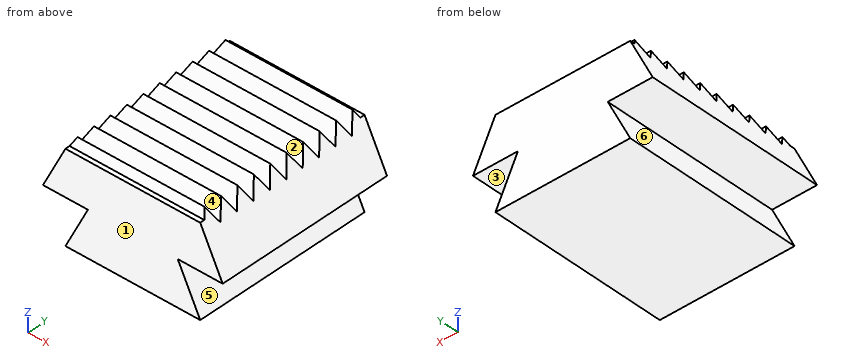
from build123d import *

# Parameters (mm, degrees)
BOSS_EXTRUDE1_DEPTH             = 5
BOSS_EXTRUDE1_DEPTH_BACK        = 5
BOSS_EXTRUDE2_REACH             = 10.66
BOSS_EXTRUDE2_DIRECTION_2_REACH = 10.66
CUT_EXTRUDE1_DEPTH              = 9.660254038
CUT_EXTRUDE1_DEPTH_BACK         = 9.660254038


with BuildPart() as part:
    # Sketch1 → Boss-Extrude1 (new, two sides: drawn at the far end of the back side and taken through both)
    with BuildSketch(Plane(origin=(0, 0, 0), x_dir=(1, 0, 0), z_dir=(0, 1, 0)).offset(-BOSS_EXTRUDE1_DEPTH_BACK)):
        Polygon((-3.75, 0), (3.75, 0), (5, 2.5), (2.5, 2.5), (3.75, 5), (-3.75, 5), (-2.5, 2.5), (-5, 2.5), align=None)
    extrude(amount=BOSS_EXTRUDE1_DEPTH + BOSS_EXTRUDE1_DEPTH_BACK)

    # Boss-Extrude2: up to this plane
    boss_extrude2_end = Plane(origin=(3.75, -5, 0), z_dir=(0.8944271909999159, 0, 0.44721359549995815))
    # Sketch3 → Boss-Extrude2 (add, up to the surface)
    with BuildSketch(Plane(origin=(0, 0, 0), x_dir=(0, 0, -1), z_dir=(1, 0, 0)), mode=Mode.PRIVATE) as boss_extrude2_sk1:
        Polygon((-0.433012702, 4.5), (0.216506351, 4.125), (0.216506351, 4.875), align=None)
    boss_extrude2_tool1 = split(extrude(boss_extrude2_sk1.sketch, amount=BOSS_EXTRUDE2_REACH, mode=Mode.PRIVATE), bisect_by=boss_extrude2_end, keep=Keep.BOTH, mode=Mode.PRIVATE)
    add(boss_extrude2_tool1.solids().sort_by_distance((0, 4.5, 0))[0])
    # Sketch3 → Boss-Extrude2 (add, up to the surface)
    with BuildSketch(Plane(origin=(0, 0, 0), x_dir=(0, 0, -1), z_dir=(1, 0, 0)), mode=Mode.PRIVATE) as boss_extrude2_sk2:
        Polygon((0.216506351, 3.875), (-0.433012702, 3.5), (0.216506351, 3.125), align=None)
    boss_extrude2_tool2 = split(extrude(boss_extrude2_sk2.sketch, amount=BOSS_EXTRUDE2_REACH, mode=Mode.PRIVATE), bisect_by=boss_extrude2_end, keep=Keep.BOTH, mode=Mode.PRIVATE)
    add(boss_extrude2_tool2.solids().sort_by_distance((0, 3.5, 0))[0])
    # Sketch3 → Boss-Extrude2 (add, up to the surface)
    with BuildSketch(Plane(origin=(0, 0, 0), x_dir=(0, 0, -1), z_dir=(1, 0, 0)), mode=Mode.PRIVATE) as boss_extrude2_sk3:
        Polygon((0.216506351, 2.875), (-0.433012702, 2.5), (0.216506351, 2.125), align=None)
    boss_extrude2_tool3 = split(extrude(boss_extrude2_sk3.sketch, amount=BOSS_EXTRUDE2_REACH, mode=Mode.PRIVATE), bisect_by=boss_extrude2_end, keep=Keep.BOTH, mode=Mode.PRIVATE)
    add(boss_extrude2_tool3.solids().sort_by_distance((0, 2.5, 0))[0])
    # Sketch3 → Boss-Extrude2 (add, up to the surface)
    with BuildSketch(Plane(origin=(0, 0, 0), x_dir=(0, 0, -1), z_dir=(1, 0, 0)), mode=Mode.PRIVATE) as boss_extrude2_sk4:
        Polygon((0.216506351, 1.875), (-0.433012702, 1.5), (0.216506351, 1.125), align=None)
    boss_extrude2_tool4 = split(extrude(boss_extrude2_sk4.sketch, amount=BOSS_EXTRUDE2_REACH, mode=Mode.PRIVATE), bisect_by=boss_extrude2_end, keep=Keep.BOTH, mode=Mode.PRIVATE)
    add(boss_extrude2_tool4.solids().sort_by_distance((0, 1.5, 0))[0])
    # Sketch3 → Boss-Extrude2 (add, up to the surface)
    with BuildSketch(Plane(origin=(0, 0, 0), x_dir=(0, 0, -1), z_dir=(1, 0, 0)), mode=Mode.PRIVATE) as boss_extrude2_sk5:
        Polygon((0.216506351, 0.875), (-0.433012702, 0.5), (0.216506351, 0.125), align=None)
    boss_extrude2_tool5 = split(extrude(boss_extrude2_sk5.sketch, amount=BOSS_EXTRUDE2_REACH, mode=Mode.PRIVATE), bisect_by=boss_extrude2_end, keep=Keep.BOTH, mode=Mode.PRIVATE)
    add(boss_extrude2_tool5.solids().sort_by_distance((0, 0.5, 0))[0])
    # Sketch3 → Boss-Extrude2 (add, up to the surface)
    with BuildSketch(Plane(origin=(0, 0, 0), x_dir=(0, 0, -1), z_dir=(1, 0, 0)), mode=Mode.PRIVATE) as boss_extrude2_sk6:
        Polygon((0.216506351, -0.125), (-0.433012702, -0.5), (0.216506351, -0.875), align=None)
    boss_extrude2_tool6 = split(extrude(boss_extrude2_sk6.sketch, amount=BOSS_EXTRUDE2_REACH, mode=Mode.PRIVATE), bisect_by=boss_extrude2_end, keep=Keep.BOTH, mode=Mode.PRIVATE)
    add(boss_extrude2_tool6.solids().sort_by_distance((0, -0.5, 0))[0])
    # Sketch3 → Boss-Extrude2 (add, up to the surface)
    with BuildSketch(Plane(origin=(0, 0, 0), x_dir=(0, 0, -1), z_dir=(1, 0, 0)), mode=Mode.PRIVATE) as boss_extrude2_sk7:
        Polygon((0.216506351, -1.125), (-0.433012702, -1.5), (0.216506351, -1.875), align=None)
    boss_extrude2_tool7 = split(extrude(boss_extrude2_sk7.sketch, amount=BOSS_EXTRUDE2_REACH, mode=Mode.PRIVATE), bisect_by=boss_extrude2_end, keep=Keep.BOTH, mode=Mode.PRIVATE)
    add(boss_extrude2_tool7.solids().sort_by_distance((0, -1.5, 0))[0])
    # Sketch3 → Boss-Extrude2 (add, up to the surface)
    with BuildSketch(Plane(origin=(0, 0, 0), x_dir=(0, 0, -1), z_dir=(1, 0, 0)), mode=Mode.PRIVATE) as boss_extrude2_sk8:
        Polygon((0.216506351, -2.125), (-0.433012702, -2.5), (0.216506351, -2.875), align=None)
    boss_extrude2_tool8 = split(extrude(boss_extrude2_sk8.sketch, amount=BOSS_EXTRUDE2_REACH, mode=Mode.PRIVATE), bisect_by=boss_extrude2_end, keep=Keep.BOTH, mode=Mode.PRIVATE)
    add(boss_extrude2_tool8.solids().sort_by_distance((0, -2.5, 0))[0])
    # Sketch3 → Boss-Extrude2 (add, up to the surface)
    with BuildSketch(Plane(origin=(0, 0, 0), x_dir=(0, 0, -1), z_dir=(1, 0, 0)), mode=Mode.PRIVATE) as boss_extrude2_sk9:
        Polygon((0.216506351, -3.125), (-0.433012702, -3.5), (0.216506351, -3.875), align=None)
    boss_extrude2_tool9 = split(extrude(boss_extrude2_sk9.sketch, amount=BOSS_EXTRUDE2_REACH, mode=Mode.PRIVATE), bisect_by=boss_extrude2_end, keep=Keep.BOTH, mode=Mode.PRIVATE)
    add(boss_extrude2_tool9.solids().sort_by_distance((0, -3.5, 0))[0])
    # Sketch3 → Boss-Extrude2 (add, up to the surface)
    with BuildSketch(Plane(origin=(0, 0, 0), x_dir=(0, 0, -1), z_dir=(1, 0, 0)), mode=Mode.PRIVATE) as boss_extrude2_sk10:
        Polygon((0.216506351, -4.125), (-0.433012702, -4.5), (0.216506351, -4.875), align=None)
    boss_extrude2_tool10 = split(extrude(boss_extrude2_sk10.sketch, amount=BOSS_EXTRUDE2_REACH, mode=Mode.PRIVATE), bisect_by=boss_extrude2_end, keep=Keep.BOTH, mode=Mode.PRIVATE)
    add(boss_extrude2_tool10.solids().sort_by_distance((0, -4.5, 0))[0])

    # Boss-Extrude2 direction 2: up to this plane
    boss_extrude2_direction_2_end = Plane(origin=(-5, -5, -2.5), z_dir=(-0.8944271909999154, 0, 0.44721359549995904))
    # Sketch3 → Boss-Extrude2 direction 2 (add, up to the surface)
    with BuildSketch(Plane(origin=(0, 0, 0), x_dir=(0, 0, -1), z_dir=(1, 0, 0)), mode=Mode.PRIVATE) as boss_extrude2_direction_2_sk1:
        Polygon((-0.433012702, 4.5), (0.216506351, 4.125), (0.216506351, 4.875), align=None)
    boss_extrude2_direction_2_tool1 = split(extrude(boss_extrude2_direction_2_sk1.sketch, amount=-BOSS_EXTRUDE2_DIRECTION_2_REACH, mode=Mode.PRIVATE), bisect_by=boss_extrude2_direction_2_end, keep=Keep.BOTH, mode=Mode.PRIVATE)
    add(boss_extrude2_direction_2_tool1.solids().sort_by_distance((0, 4.5, 0))[0])
    # Sketch3 → Boss-Extrude2 direction 2 (add, up to the surface)
    with BuildSketch(Plane(origin=(0, 0, 0), x_dir=(0, 0, -1), z_dir=(1, 0, 0)), mode=Mode.PRIVATE) as boss_extrude2_direction_2_sk2:
        Polygon((0.216506351, 3.875), (-0.433012702, 3.5), (0.216506351, 3.125), align=None)
    boss_extrude2_direction_2_tool2 = split(extrude(boss_extrude2_direction_2_sk2.sketch, amount=-BOSS_EXTRUDE2_DIRECTION_2_REACH, mode=Mode.PRIVATE), bisect_by=boss_extrude2_direction_2_end, keep=Keep.BOTH, mode=Mode.PRIVATE)
    add(boss_extrude2_direction_2_tool2.solids().sort_by_distance((0, 3.5, 0))[0])
    # Sketch3 → Boss-Extrude2 direction 2 (add, up to the surface)
    with BuildSketch(Plane(origin=(0, 0, 0), x_dir=(0, 0, -1), z_dir=(1, 0, 0)), mode=Mode.PRIVATE) as boss_extrude2_direction_2_sk3:
        Polygon((0.216506351, 2.875), (-0.433012702, 2.5), (0.216506351, 2.125), align=None)
    boss_extrude2_direction_2_tool3 = split(extrude(boss_extrude2_direction_2_sk3.sketch, amount=-BOSS_EXTRUDE2_DIRECTION_2_REACH, mode=Mode.PRIVATE), bisect_by=boss_extrude2_direction_2_end, keep=Keep.BOTH, mode=Mode.PRIVATE)
    add(boss_extrude2_direction_2_tool3.solids().sort_by_distance((0, 2.5, 0))[0])
    # Sketch3 → Boss-Extrude2 direction 2 (add, up to the surface)
    with BuildSketch(Plane(origin=(0, 0, 0), x_dir=(0, 0, -1), z_dir=(1, 0, 0)), mode=Mode.PRIVATE) as boss_extrude2_direction_2_sk4:
        Polygon((0.216506351, 1.875), (-0.433012702, 1.5), (0.216506351, 1.125), align=None)
    boss_extrude2_direction_2_tool4 = split(extrude(boss_extrude2_direction_2_sk4.sketch, amount=-BOSS_EXTRUDE2_DIRECTION_2_REACH, mode=Mode.PRIVATE), bisect_by=boss_extrude2_direction_2_end, keep=Keep.BOTH, mode=Mode.PRIVATE)
    add(boss_extrude2_direction_2_tool4.solids().sort_by_distance((0, 1.5, 0))[0])
    # Sketch3 → Boss-Extrude2 direction 2 (add, up to the surface)
    with BuildSketch(Plane(origin=(0, 0, 0), x_dir=(0, 0, -1), z_dir=(1, 0, 0)), mode=Mode.PRIVATE) as boss_extrude2_direction_2_sk5:
        Polygon((0.216506351, 0.875), (-0.433012702, 0.5), (0.216506351, 0.125), align=None)
    boss_extrude2_direction_2_tool5 = split(extrude(boss_extrude2_direction_2_sk5.sketch, amount=-BOSS_EXTRUDE2_DIRECTION_2_REACH, mode=Mode.PRIVATE), bisect_by=boss_extrude2_direction_2_end, keep=Keep.BOTH, mode=Mode.PRIVATE)
    add(boss_extrude2_direction_2_tool5.solids().sort_by_distance((0, 0.5, 0))[0])
    # Sketch3 → Boss-Extrude2 direction 2 (add, up to the surface)
    with BuildSketch(Plane(origin=(0, 0, 0), x_dir=(0, 0, -1), z_dir=(1, 0, 0)), mode=Mode.PRIVATE) as boss_extrude2_direction_2_sk6:
        Polygon((0.216506351, -0.125), (-0.433012702, -0.5), (0.216506351, -0.875), align=None)
    boss_extrude2_direction_2_tool6 = split(extrude(boss_extrude2_direction_2_sk6.sketch, amount=-BOSS_EXTRUDE2_DIRECTION_2_REACH, mode=Mode.PRIVATE), bisect_by=boss_extrude2_direction_2_end, keep=Keep.BOTH, mode=Mode.PRIVATE)
    add(boss_extrude2_direction_2_tool6.solids().sort_by_distance((0, -0.5, 0))[0])
    # Sketch3 → Boss-Extrude2 direction 2 (add, up to the surface)
    with BuildSketch(Plane(origin=(0, 0, 0), x_dir=(0, 0, -1), z_dir=(1, 0, 0)), mode=Mode.PRIVATE) as boss_extrude2_direction_2_sk7:
        Polygon((0.216506351, -1.125), (-0.433012702, -1.5), (0.216506351, -1.875), align=None)
    boss_extrude2_direction_2_tool7 = split(extrude(boss_extrude2_direction_2_sk7.sketch, amount=-BOSS_EXTRUDE2_DIRECTION_2_REACH, mode=Mode.PRIVATE), bisect_by=boss_extrude2_direction_2_end, keep=Keep.BOTH, mode=Mode.PRIVATE)
    add(boss_extrude2_direction_2_tool7.solids().sort_by_distance((0, -1.5, 0))[0])
    # Sketch3 → Boss-Extrude2 direction 2 (add, up to the surface)
    with BuildSketch(Plane(origin=(0, 0, 0), x_dir=(0, 0, -1), z_dir=(1, 0, 0)), mode=Mode.PRIVATE) as boss_extrude2_direction_2_sk8:
        Polygon((0.216506351, -2.125), (-0.433012702, -2.5), (0.216506351, -2.875), align=None)
    boss_extrude2_direction_2_tool8 = split(extrude(boss_extrude2_direction_2_sk8.sketch, amount=-BOSS_EXTRUDE2_DIRECTION_2_REACH, mode=Mode.PRIVATE), bisect_by=boss_extrude2_direction_2_end, keep=Keep.BOTH, mode=Mode.PRIVATE)
    add(boss_extrude2_direction_2_tool8.solids().sort_by_distance((0, -2.5, 0))[0])
    # Sketch3 → Boss-Extrude2 direction 2 (add, up to the surface)
    with BuildSketch(Plane(origin=(0, 0, 0), x_dir=(0, 0, -1), z_dir=(1, 0, 0)), mode=Mode.PRIVATE) as boss_extrude2_direction_2_sk9:
        Polygon((0.216506351, -3.125), (-0.433012702, -3.5), (0.216506351, -3.875), align=None)
    boss_extrude2_direction_2_tool9 = split(extrude(boss_extrude2_direction_2_sk9.sketch, amount=-BOSS_EXTRUDE2_DIRECTION_2_REACH, mode=Mode.PRIVATE), bisect_by=boss_extrude2_direction_2_end, keep=Keep.BOTH, mode=Mode.PRIVATE)
    add(boss_extrude2_direction_2_tool9.solids().sort_by_distance((0, -3.5, 0))[0])
    # Sketch3 → Boss-Extrude2 direction 2 (add, up to the surface)
    with BuildSketch(Plane(origin=(0, 0, 0), x_dir=(0, 0, -1), z_dir=(1, 0, 0)), mode=Mode.PRIVATE) as boss_extrude2_direction_2_sk10:
        Polygon((0.216506351, -4.125), (-0.433012702, -4.5), (0.216506351, -4.875), align=None)
    boss_extrude2_direction_2_tool10 = split(extrude(boss_extrude2_direction_2_sk10.sketch, amount=-BOSS_EXTRUDE2_DIRECTION_2_REACH, mode=Mode.PRIVATE), bisect_by=boss_extrude2_direction_2_end, keep=Keep.BOTH, mode=Mode.PRIVATE)
    add(boss_extrude2_direction_2_tool10.solids().sort_by_distance((0, -4.5, 0))[0])

    # Sketch4 → Cut-Extrude1 (cut, two sides: drawn at the far end of the back side and taken through both)
    with BuildSketch(Plane(origin=(0, 0, 0), x_dir=(0, 0, -1), z_dir=(1, 0, 0)).offset(-CUT_EXTRUDE1_DEPTH_BACK)):
        Polygon((0.433012702, 4), (-0.216506351, 4.375), (-0.216506351, 3.625), align=None)
        Polygon((-0.216506351, 2.625), (0.433012702, 3), (-0.216506351, 3.375), align=None)
        Polygon((-0.216506351, 1.625), (0.433012702, 2), (-0.216506351, 2.375), align=None)
        Polygon((-0.216506351, 0.625), (0.433012702, 1), (-0.216506351, 1.375), align=None)
        Polygon((-0.216506351, -0.375), (0.433012702, 0), (-0.216506351, 0.375), align=None)
        Polygon((-0.216506351, -1.375), (0.433012702, -1), (-0.216506351, -0.625), align=None)
        Polygon((-0.216506351, -2.375), (0.433012702, -2), (-0.216506351, -1.625), align=None)
        Polygon((-0.216506351, -3.375), (0.433012702, -3), (-0.216506351, -2.625), align=None)
        Polygon((-0.216506351, -4.375), (0.433012702, -4), (-0.216506351, -3.625), align=None)
    extrude(amount=CUT_EXTRUDE1_DEPTH + CUT_EXTRUDE1_DEPTH_BACK, mode=Mode.SUBTRACT)


solid = part.part
Design review of the part built by this model. Coordinates are the model's own, in mm. Face numbers are marked on the shaded views. A direction names the side the tool comes from. Coordinates: 2 decimals unless noted, no trailing zeros. Loops run counter-clockwise (first coordinate to the right, second up) from the corner with the lowest first, then second, coordinate; pieces in that order, holes last. Notation, with made-up numbers: (-29.75, -30.75) -> (14.25, -30.75) arc R12 cw to (14.25, -7.75) -> close; hole circle Ø1 at (-30, 39.5). An arc over 180 degrees is marked (long way). Use a Markdown table: item, result. Add a question column.
Item 1: We need section C-C, the plane z = -4.1. Write out the cut boundary in (x, y).
Item 2: Clearance check with a flat-ended pin moving along its axis: P1, Ø3, axis at y = -2.5, z = -3, coming from the -X side. State where the tip first meets the part, or that it passes through.
Item 3: The part is to be moulded in two halves that separate along Z. For the marked faces 1, 2 and 3, say which applies: +Z half, -Z half, draft (parallel to the pull), parting line (faces both ways), or undercut.
Item 4: Machinability: for the marked faces 4, 5 and 6, which of the approach directions +Z, -Z, +X, -X, +Y, -Y give a long, thin tool a straight path to every point of the face, cutting with its end or side? Answer none if there is none.
Item 5: Wall thickness on L1, parallel to Z at x = -3.5, y = 4.25; L2, parallel to Z at x = -1, y = 1.75; L3, parallel to Z at x = 4, y = -1: over which ranges is each line inside the solid? List them lowest first. Write a range as from..to.
Item 6: We need section B-B, the plane y = -0.25. Write out the cut boundary in (x, z).
Item 7: We need section D-D, the plane x = 0.75. Write out the cut boundary in (y, z), and give its area (3 significant figures).
Numbers:
| question | item | result |
|---|---|---|
| 1 | outline | (-3.3, -5) -> (3.3, -5) -> (3.3, 5) -> (-3.3, 5) -> close |
| 2 | P1 | stops at x = -5 |
| 3 | face 1 | draft |
| 3 | face 2 | +Z half |
| 3 | face 3 | undercut |
| 4 | face 4 | +Z, +X, -X |
| 4 | face 5 | +X, +Y, -Y |
| 4 | face 6 | -X, +Y, -Y |
| 5 | L1 | z = -5..-4.5, -2.5..0 |
| 5 | L2 | z = -5..0 |
| 5 | L3 | z = -2.5..-0.5 |
| 6 | outline | (-5, -2.5) -> (-2.5, -2.5) -> (-3.75, -5) -> (3.75, -5) -> (2.5, -2.5) -> (5, -2.5) -> (3.75, 0) -> (-3.75, 0) -> close |
| 7 | outline | (-5, -5) -> (5, -5) -> (5, 0) -> (4.75, 0) -> (4.5, 0.43) -> (4, -0.43) -> (3.5, 0.43) -> (3, -0.43) -> (2.5, 0.43) -> (2, -0.43) -> (1.5, 0.43) -> (1, -0.43) -> (0.5, 0.43) -> (0, -0.43) -> (-0.5, 0.43) -> (-1, -0.43) -> (-1.5, 0.43) -> (-2, -0.43) -> (-2.5, 0.43) -> (-3, -0.43) -> (-3.5, 0.43) -> (-4, -0.43) -> (-4.5, 0.43) -> (-4.75, 0) -> (-5, 0) -> close |
| 7 | area | 50.1 mm^2 |
